Model file for the job. Use its own axes, mm. Face numbers are marked on the shaded views. Coordinates: 2 decimals unless noted, no trailing zeros. Loops run counter-clockwise (first coordinate to the right, second up) from the corner with the lowest first, then second, coordinate; pieces in that order, holes last. Notation, with made-up numbers: (59.5, 7) -> (115.5, 7) arc R26 ccw to (115.5, 38) -> close; hole circle Ø9 at (-38.75, -5.5). An arc over 180 degrees is marked (long way). Use one line per item in the form item = value.
```python
from build123d import *

# Parameters (mm, degrees)
CUT_EXTRUDE_1_DEPTH = 1


with BuildPart() as part:
    # 草圖2 → 旋轉1 (revolve)
    with BuildSketch(Plane.XY):
        with BuildLine():
            Line((0, 0), (1.5, 0))
            Line((1.5, 0), (1.5, 20))
            Line((1.5, 20), (2.3, 20))
            Line((2.3, 20), (2.3, 20.6))
            ThreePointArc((2.3, 20.6), (2.007106781, 21.307106781), (1.3, 21.6))
            Line((1.3, 21.6), (0, 21.6))
            Line((0, 21.6), (0, 0))
        make_face()
    revolve(axis=Axis((0, 21.6, 0), (0, -1, 0)))

    # 草圖3 → 除料-伸長1 (cut)
    with BuildSketch(Plane(origin=(0, 21.6, 0), x_dir=(1, 0, 0), z_dir=(0, 1, 0))):
        Polygon((-0.257139239, 0.26020042), (-0.257139239, 1.063618051), (0.311378397, 1.063618051), (0.311378397, 0.26020042), (1.022434592, 0.26020042), (1.022434592, -0.285133973), (0.311378397, -0.285133973), (0.311378397, -1.013251047), (-0.257139239, -1.013251047), (-0.257139239, -0.285133973), (-1.016312229, -0.285133973), (-1.016312229, 0.26020042), align=None)
    extrude(amount=-CUT_EXTRUDE_1_DEPTH, mode=Mode.SUBTRACT)


solid = part.part
```
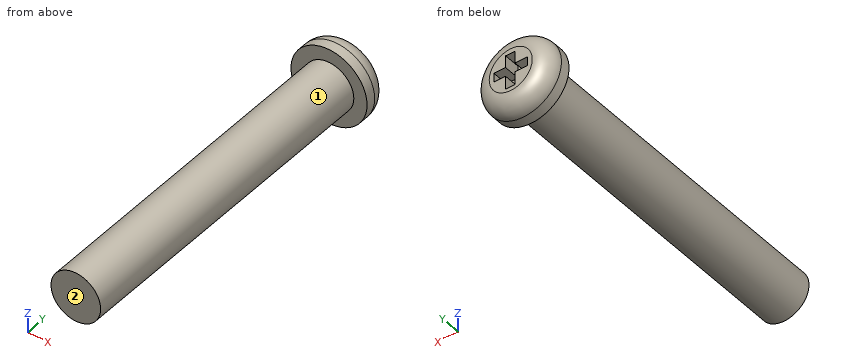
Q1. Pin check, flat tips, straight feed: pin 1 Ø0.6 at (y, z) = (21, -1) entering from -X; pin 2 Ø0.6 at (y, z) = (21.5, -1) entering from +X; pin 3 Ø0.8 at (x, y) = (0.5, 21.5) entering from -Z. Stop position of each tip, or through.
Result:
pin_1 = -2.14
pin_2 = 1.89
pin_3 = -2.12
Q2. Band-saw the part on C-C, the plane y = 14. Write the cut outline in (x, z).
Result:
outline = circle Ø3 at (0, 0)
Q3. Band-saw the part on B-B, the plane x = 0. Write the cut outline in (y, z), and give its area (3 significant figures).
Result:
outline = (0, -1.5) -> (20, -1.5) -> (20, -2.3) -> (20.6, -2.3) arc R1 ccw to (21.6, -1.3) -> (21.6, -1.06) -> (20.6, -1.06) -> (20.6, 1.01) -> (21.6, 1.01) -> (21.6, 1.3) arc R1 ccw to (20.6, 2.3) -> (20, 2.3) -> (20, 1.5) -> (0, 1.5) -> close
area = 64.9 mm2
Q4. Band-saw the part on A-A, the plane z = 0. Write the cut outline in (x, y).
Result:
outline = (-2.3, 20) -> (-1.5, 20) -> (-1.5, 0) -> (1.5, 0) -> (1.5, 20) -> (2.3, 20) -> (2.3, 20.6) arc R1 ccw to (1.3, 21.6) -> (1.02, 21.6) -> (1.02, 20.6) -> (-1.02, 20.6) -> (-1.02, 21.6) -> (-1.3, 21.6) arc R1 ccw to (-2.3, 20.6) -> close
Q5. Wall check: line 1 along X through (y, z) = (13.5, -1.1); line 2 along Z through (x, y) = (-0.1, 12.25). Give the ranges that are in metal, low to high.
Result:
line_1 = -1.02 to 1.02
line_2 = -1.5 to 1.5
Q6. Mould opens along X. For the marked faces 1 and 2 say: released by +X, released by -X, zero draft, split by the parting line, or undercut.
Result:
face_1 = split by the parting line
face_2 = zero draft
